```python
from build123d import *

# Parameters (mm, degrees)
CROQUIS1_W              = 105
CROQUIS1_H              = 10
CROQUIS1_W_2            = 5
CROQUIS1_H_2            = 33.5
SALIENTE_EXTRUIR1_DEPTH = 10
CROQUIS2_R              = 3.2
CORTAR_EXTRUIR1_DEPTH   = 111.759992767
CROQUIS3_R              = 1.95
CORTAR_EXTRUIR2_DEPTH   = 4.9
CROQUIS4_R              = 1.65
CORTAR_EXTRUIR3_DEPTH   = 115.406232338
REDONDEO1_R             = 3
CROQUIS7_R              = 1.65
SALIENTE_EXTRUIR2_DEPTH = 10


with BuildPart() as part:
    # Croquis1 → Saliente-Extruir1 (new body)
    with BuildSketch(Plane.XY):
        with Locations((10.314275766, 87)):
            Rectangle(CROQUIS1_W, CROQUIS1_H)
        with Locations((65.314275766, 87)):
            Rectangle(CROQUIS1_W_2, CROQUIS1_H)
        with Locations((65.314275766, 65.25)):
            Rectangle(CROQUIS1_W_2, CROQUIS1_H_2)
        with Locations((65.314275766, 31.75)):
            Rectangle(CROQUIS1_W_2, CROQUIS1_H_2)
        with Locations((65.314275766, 10)):
            Rectangle(CROQUIS1_W_2, CROQUIS1_H)
        with Locations((10.314275766, 10)):
            Rectangle(CROQUIS1_W, CROQUIS1_H)
    extrude(amount=SALIENTE_EXTRUIR1_DEPTH)

    # Croquis2 → Cortar-Extruir1 (cut, through all)
    with BuildSketch(Plane(origin=(0, 92, 0), x_dir=(1, 0, 0), z_dir=(0, 1, 0))):
        with Locations(Location((55.860494793, -5, 0), (0, 0, 180))):
            Circle(CROQUIS2_R)
        with BuildLine():
            Line((12.425652442, -8.2), (-27.574347558, -8.2))
            ThreePointArc((-27.574347558, -8.2), (-30.774347558, -5), (-27.574347558, -1.8))
            Line((-27.574347558, -1.8), (12.425652442, -1.8))
            ThreePointArc((12.425652442, -1.8), (15.625652442, -5), (12.425652442, -8.2))
        make_face()
    extrude(amount=-CORTAR_EXTRUIR1_DEPTH, mode=Mode.SUBTRACT)

    # Croquis3 → Cortar-Extruir2 (cut)
    with BuildSketch(Plane.XY.offset(10)):
        with Locations((-36.979834841, 87)):
            Circle(CROQUIS3_R)
        with Locations((-36.979834841, 10)):
            Circle(CROQUIS3_R)
        with Locations((43.869300962, 10)):
            Circle(CROQUIS3_R)
        with Locations((43.869300962, 87)):
            Circle(CROQUIS3_R)
    extrude(amount=-CORTAR_EXTRUIR2_DEPTH, mode=Mode.SUBTRACT)

    # Croquis4 → Cortar-Extruir3 (cut, through all)
    with BuildSketch(Plane.XY.offset(5.1)):
        with Locations((-36.979834841, 87)):
            Circle(CROQUIS4_R)
        with Locations((-36.979834841, 10)):
            Circle(CROQUIS4_R)
        with Locations((43.869300962, 10)):
            Circle(CROQUIS4_R)
        with Locations((43.869300962, 87)):
            Circle(CROQUIS4_R)
    extrude(amount=-CORTAR_EXTRUIR3_DEPTH, mode=Mode.SUBTRACT)

    # Redondeo1
    redondeo1_edges = [part.edges().sort_by_distance(p)[0] for p in [
        (-42.185724234, 82, 5),
        (-42.185724234, 92, 5),
        (67.814275766, 92, 5),
        (67.814275766, 5, 5),
        (-42.185724234, 5, 5),
        (-42.185724234, 15, 5),
    ]]
    fillet(redondeo1_edges, radius=REDONDEO1_R)

    # Croquis7 → Saliente-Extruir2 (add)
    with BuildSketch(Plane(origin=(0, 0, 0), x_dir=(-1, 0, 0), z_dir=(0, 0, -1))):
        with BuildLine():
            Line((39.185724234, 92), (-64.814275766, 92))
            ThreePointArc((-64.814275766, 92), (-66.93559611, 91.121320344), (-67.814275766, 89))
            Line((-67.814275766, 89), (-67.814275766, 8))
            ThreePointArc((-67.814275766, 8), (-66.93559611, 5.878679656), (-64.814275766, 5))
            Line((-64.814275766, 5), (39.185724234, 5))
            ThreePointArc((39.185724234, 5), (41.307044577, 5.878679656), (42.185724234, 8))
            Line((42.185724234, 8), (42.185724234, 12))
            ThreePointArc((42.185724234, 12), (41.307044577, 14.121320344), (39.185724234, 15))
            Line((39.185724234, 15), (-62.814275766, 15))
            Line((-62.814275766, 15), (-62.814275766, 82))
            Line((-62.814275766, 82), (39.185724234, 82))
            ThreePointArc((39.185724234, 82), (41.307044577, 82.878679656), (42.185724234, 85))
            Line((42.185724234, 85), (42.185724234, 89))
            ThreePointArc((42.185724234, 89), (41.307044577, 91.121320344), (39.185724234, 92))
        make_face()
        with Locations(Location((36.979834841, 87, 0), (0, 0, 180))):
            Circle(CROQUIS7_R, mode=Mode.SUBTRACT)
        with Locations(Location((36.979834841, 10, 0), (0, 0, 180))):
            Circle(CROQUIS7_R, mode=Mode.SUBTRACT)
        with Locations(Location((-43.869300962, 10, 0), (0, 0, 180))):
            Circle(CROQUIS7_R, mode=Mode.SUBTRACT)
        with Locations(Location((-43.869300962, 87, 0), (0, 0, 180))):
            Circle(CROQUIS7_R, mode=Mode.SUBTRACT)
    extrude(amount=SALIENTE_EXTRUIR2_DEPTH)


solid = part.part
```
Geometry: final body of the model. Coordinates: model frame, mm. A direction names the side the tool comes from. Round coordinates to 2 decimals unless told otherwise and drop trailing zeros. Order: outer loops, then holes, each group sorted by start corner. A loop starts at its lowest first (then second) coordinate and runs counter-clockwise, first axis right, second up. Notation, with made-up numbers: (8, 80) - (37, 80) arc R24 cw to (37, 92) - close; hole circle Ø6 at (27.25, 41). An arc over 180 degrees is marked (long way). Use CSV: the item, a comma, the result in double quotes. Start each with the question number.
Q1. Access query for faces 5 (the face through (44.631, 88.464, -2.344)), 6 (the face through (15.625, 10.07, 4.93)), 7 (the face through (13, 82, 0)). Directions: +Z, -Z, +X, -X, +Y, -Y. A direction counts if a zero-diameter tool reaches every point of the face in a straight line with its end or side. Return the directions, or none.
Q2. Section query D-D (y = 54). Return loops of the section in (x, z), and give its area (3 significant figures).
Q3. Material intervals for line 1 along Y through (x, z) = (41.5, 5.75); line 2 along Y through (x, z) = (-37, -6.75); line 3 along X through (y, z) = (32, -4), sorted ascending. Write a range as from..to.
Q4. Section query A-A (y = 87). Return loops of the section in (x, z), and give its area (3 significant figures).
Q5. Section query B-B (x = 39). Return loops of the section in (y, z), and give its area (3 significant figures).
Q6. Mould query, pull axis Z, two halves, no side actions, for faces 1 (the face through (15.625, 87.07, 4.93)), 2 (the face through (-30.774, 87.07, 5.07)), 3 (the face through (17, 13, -10)), 4 (the face through (45.67, 9.25, 7.58)). Classes: +Z half, -Z half, draft (parallel to the pull), parting line (faces both ways), or undercut.
Q7. Section query C-C (x = 3). Return loops of the section in (y, z).
Q8. First-contact query: pin 1 (12 mm diameter, centred on y = 62.5, z = -5.5, fed in from -X). Flat tip, straight axial feed; report the tip coordinate or a pass-through.
Result set:
1,face 5,"+Z, -Z"
1,face 6,"+Y, -Y"
1,face 7,"+Z, -Z, -X"
2,outline,"(62.81, -10) - (67.81, -10) - (67.81, 10) - (62.81, 10) - close"
2,area,"100 mm2"
3,line 1,"y = 5..15, 82..92"
3,line 2,"y = 5..8.35, 11.65..15, 82..85.35, 88.65..92"
3,line 3,"x = 62.81..67.81"
4,outline,"(-42.19, -10) - (-38.63, -10) - (-38.63, 5.1) - (-38.93, 5.1) - (-38.93, 10) - (-42.19, 10) - close; (-35.33, -10) - (42.22, -10) - (42.22, 5.1) - (41.92, 5.1) - (41.92, 10) - (-35.03, 10) - (-35.03, 5.1) - (-35.33, 5.1) - close; (45.52, -10) - (67.81, -10) - (67.81, 10) - (45.82, 10) - (45.82, 5.1) - (45.52, 5.1) - close; hole (-27.57, 1.8) - (12.43, 1.8) arc R3.2 ccw to (12.43, 8.2) - (-27.57, 8.2) arc R3.2 ccw to start; hole circle Ø6.4 at (55.86, 5)"
4,area,"1,740 mm2"
5,outline,"(5, -10) - (15, -10) - (15, 10) - (5, 10) - close; (82, -10) - (92, -10) - (92, 10) - (82, 10) - close"
5,area,"400 mm2"
6,face 1,"undercut"
6,face 2,"undercut"
6,face 3,"-Z half"
6,face 4,"draft"
7,outline,"(5, -10) - (15, -10) - (15, 1.8) - (5, 1.8) - close; (5, 8.2) - (15, 8.2) - (15, 10) - (5, 10) - close; (82, -10) - (92, -10) - (92, 1.8) - (82, 1.8) - close; (82, 8.2) - (92, 8.2) - (92, 10) - (82, 10) - close"
8,pin 1,"stops at x = 62.81"
